Study the drawing (mm; zero at the part's minimum x, y, z) and answer. A direction names the side the tool comes from. Round coordinates to 2 decimals unless told otherwise and drop trailing zeros. Write each loop counter-clockwise with the first axis right and the second up, starting at its lowest first coordinate (ties: lowest second). Pieces come first, ordered by that corner, then holes.
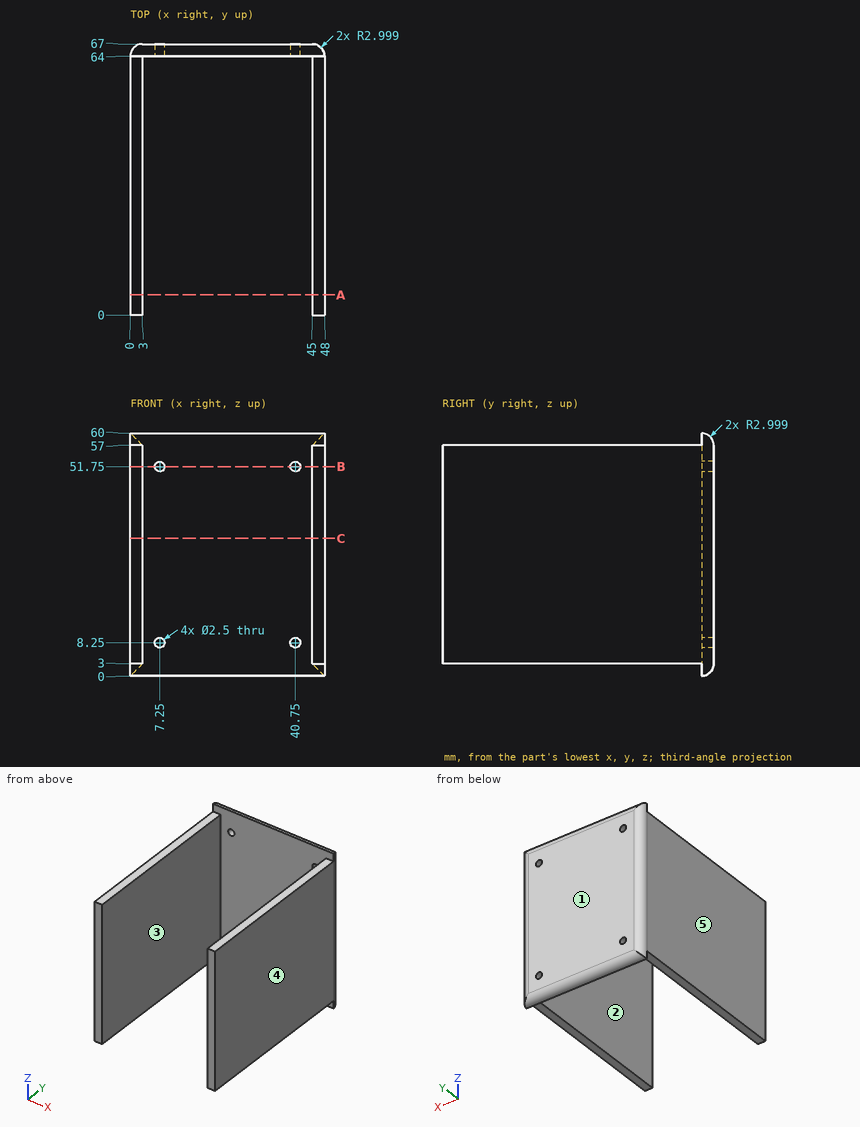
Q1. Given pin 1 (3 mm diameter, centred on x = 7.25, z = 51.75, fed in from -Y); pin 2 (1.5 mm diameter, centred on x = 1, y = 30.5, fed in from -Z); pin 3 (2 mm diameter, centred on x = 40.75, z = 51.75, fed in from +Y); pin 4 (2.5 mm diameter, centred on x = 47, y = 37, fed in from +Z), each flat-ended and moving along its own axis, determine where each tip first touches the part or whether it passes through.
Q2. Find section C-C (z = 34). Determine the outline of the cut face in (x, y).
Q3. The mould has two halves that part along X. Classify the marked faces 3, 4 and 5: +X half, -X half, draft (parallel to the pull), parting line (faces both ways), or undercut.
Q4. Find the intervals of material crossed by L1, parallel to X at y = 19, z = 51; L2, parallel to Y at x = 21, z = 29; L3, parallel to X at y = 65, z = 51, in increasing order.
Q5. Find section A-A (y = 5). Determine the outline of the cut face in (x, z).
Q6. Find section B-B (z = 51.75). Determine the outline of the cut face in (x, y), plus the area to 3 significant figures.
Q7. A tool of negligible diameter and unlimited length cuts with its end or side. For the marked faces 1 and 2, from which of +Z, -Z, +X, -X, +Y, -Y can it reach the whole face along a straight path? Write none if from no direction.
Report:
1. pin 1: stops at y = 64
1. pin 2: stops at z = 3
1. pin 3: passes through
1. pin 4: stops at z = 57
2. outline: (0, 0) - (3, 0) - (3, 64) - (45, 64) - (45, 0) - (48, 0) - (48, 64) arc R3 ccw to (45, 67) - (3, 67) arc R3 ccw to (0, 64) - close
3. face 3: undercut
3. face 4: +X half
3. face 5: -X half
4. L1: x = 0 to 3, 45 to 48
4. L2: y = 64 to 67
4. L3: x = 0.17 to 6.25, 8.25 to 39.75, 41.75 to 47.83
5. outline: (0, 3) - (3, 3) - (3, 57) - (0, 57) - close; (45, 3) - (48, 3) - (48, 57) - (45, 57) - close
6. outline: (0, 0) - (3, 0) - (3, 64) - (6, 64) - (6, 67) - (3, 67) arc R3 ccw to (0, 64) - close; (8.5, 64) - (39.5, 64) - (39.5, 67) - (8.5, 67) - close; (42, 64) - (45, 64) - (45, 0) - (48, 0) - (48, 64) arc R3 ccw to (45, 67) - (42, 67) - close
6. area: 509 mm2
7. face 1: +Z, -Z, +X, -X, +Y
7. face 2: +Z, -Z, -Y
